Check sheet for the modelled part. Datum: model origin and axes. Units: mm. A direction names the side the tool comes from. Round coordinates to 2 decimals unless told otherwise and drop trailing zeros. Order: outer loops, then holes, each group sorted by start corner. A loop starts at its lowest first (then second) coordinate and runs counter-clockwise, first axis right, second up. Notation, with made-up numbers: (17.5, 50.5) -> (55.5, 50.5) arc R29 ccw to (55.5, 73.5) -> close; hole circle Ø11 at (35, -31.75). An arc over 180 degrees is marked (long way). Answer in a Markdown table with one row per item. Add a question column.
1. Access from +Z, -Z, +X, -X, +Y, -Y to the whole of each face (thin tool, end or side, straight path). Record for faces 4 (the flat face through (-10, -73, 12)), 5 (the flat face through (-50, -57, -5)), 6 (the flat face through (-18, -39, -15)), 7 (the flat face through (-80, -39, -7)), 8 (the flat face through (-55, -39, -17)).
2. Sectioned sample at A-A, the plane y = -55. Record the boundary of the cut face in (x, z), then the cut area to 3 significant figures.
3. Sectioned sample at C-C, the plane y = -38. Record the boundary of the cut face in (x, z).
4. Draft check along X on faces 1 (the flat face through (-68, -39, -15)), 2 (the flat face through (-60, -7, 7)), 3 (the cylindrical face through (-53, -61, -2)). Enter one of: +X half, -X half, draft (parallel to the pull), parting line (faces both ways), or undercut.
5. Material ranges on L1, parallel to Y at x = -45, z = -2; L2, parallel to Y at x = -45, z = -10.25; L3, parallel to Z at x = -61, y = -44, recorded low to high. Write a range as from..to.
6. Depth check by flat-ended pin: P1, Ø1.5, axis at y = -51, z = 15, coming from the -X side; P2, Ø11.5, axis at x = -45, y = -55, coming from the +Z side; P3, Ø5.5, axis at y = -21.5, z = -18.5, coming from the +X side. Enter the tip coordinate at first touch or a pass-through.
7. Sectioned sample at D-D, the plane x = -11. Record the boundary of the cut face in (y, z).
8. Sectioned sample at B-B, the plane x = -45. Record the boundary of the cut face in (y, z), then the cut area to 3 significant figures.
```python
from build123d import *

# Parameters (mm, degrees)
F1_DEPTH  = 80
F2_W      = 10
F2_H      = 25
F3_DEPTH  = 80
F5_DEPTH  = 25
F7_DEPTH  = 25
F9_DEPTH  = 80.001
F10_R     = 10
F11_DEPTH = 5
F12_R     = 5
F13_DEPTH = 25


with BuildPart() as f1:
    # F0 (on Front) → F1 (new body)
    with BuildSketch(Plane.XZ):
        Polygon((0, -15), (0, 0), (-80, 0), (-80, -15), (-55, -15), (-55, -20), (-35, -20), (-35, -15), align=None)
    extrude(amount=F1_DEPTH)

    # F2 (on face) → F3 (join)
    with BuildSketch(Plane.XZ.offset(80)):
        with Locations((-5, 12.5)):
            Rectangle(F2_W, F2_H)
    extrude(amount=-F3_DEPTH)

    # F4 (on face) → F5 (join, through all)
    with BuildSketch(Plane.XY.offset(25)):
        Polygon((-50, -25), (-10, -65), (-10, -25), align=None)
    extrude(amount=-F5_DEPTH)

    # F6 (on face) → F7 (join)
    with BuildSketch(Plane.XY):
        Polygon((-60, -15), (-50, -25), (-10, -25), (-10, 0), (-60, 0), align=None)
    extrude(amount=F7_DEPTH)

    # F8 (on face) → F9 (cut, through all)
    with BuildSketch(Plane.YZ):
        Polygon((0, 10.566243), (0, 25), (-25, 25), align=None)
    extrude(amount=-F9_DEPTH, mode=Mode.SUBTRACT)

    # F10 (on face) → F11 (cut)
    with BuildSketch(Plane.XY):
        with Locations((-45, -55)):
            Circle(F10_R)
    extrude(amount=-F11_DEPTH, mode=Mode.SUBTRACT)

    # F12 (on face) → F13 (cut)
    with BuildSketch(Plane.XY.offset(-5)):
        with Locations((-45, -55)):
            Circle(F12_R)
    extrude(amount=-F13_DEPTH, mode=Mode.SUBTRACT)


solid = f1.part
```
Answer key:
| question | item | result |
|---|---|---|
| 1 | face 4 | +Z, -X, -Y |
| 1 | face 5 | +Z |
| 1 | face 6 | -Z, +X, +Y, -Y |
| 1 | face 7 | +Z, -Z, -X, +Y, -Y |
| 1 | face 8 | -Z, -X, +Y, -Y |
| 2 | outline | (-80, -15) -> (-55, -15) -> (-55, -20) -> (-50, -20) -> (-50, -5) -> (-55, -5) -> (-55, 0) -> (-80, 0) -> close; (-40, -20) -> (-35, -20) -> (-35, -15) -> (0, -15) -> (0, 25) -> (-20, 25) -> (-20, 0) -> (-35, 0) -> (-35, -5) -> (-40, -5) -> close |
| 2 | area | 1,550 mm² |
| 3 | outline | (-80, -15) -> (-55, -15) -> (-55, -20) -> (-35, -20) -> (-35, -15) -> (0, -15) -> (0, 25) -> (-37, 25) -> (-37, 0) -> (-80, 0) -> close |
| 4 | face 1 | draft |
| 4 | face 2 | -X half |
| 4 | face 3 | undercut |
| 5 | L1 | y = -80..-65, -45..0 |
| 5 | L2 | y = -80..-60, -50..0 |
| 5 | L3 | z = -15..0 |
| 6 | P1 | stops at x = -24.75 |
| 6 | P2 | stops at z = -5 |
| 6 | P3 | stops at x = -35 |
| 7 | outline | (-80, -15) -> (0, -15) -> (0, 10.57) -> (-25, 25) -> (-64, 25) -> (-64, 0) -> (-80, 0) -> close |
| 8 | outline | (-80, -20) -> (-60, -20) -> (-60, -5) -> (-65, -5) -> (-65, 0) -> (-80, 0) -> close; (-50, -20) -> (0, -20) -> (0, 10.57) -> (-25, 25) -> (-30, 25) -> (-30, 0) -> (-45, 0) -> (-45, -5) -> (-50, -5) -> close |
| 8 | area | 1,920 mm² |
